Answer from the drawing. Dimensions are ordinates in mm from the lowest x, y and z of the part. A direction names the side the tool comes from. Give positions to 0.01 mm unless a question says otherwise; leave off trailing zeros. Order: outer loops, then holes, each group sorted by start corner. A loop starts at its lowest first (then second) coordinate and runs counter-clockwise, first axis right, second up. Notation, with made-up numbers: (67, 73) - (89, 73) arc R20 ccw to (89, 99) - close; hole circle Ø1 at (29, 25). An arc over 180 degrees is marked (long way). Answer in a Markdown table with one row per item. Add a question column.
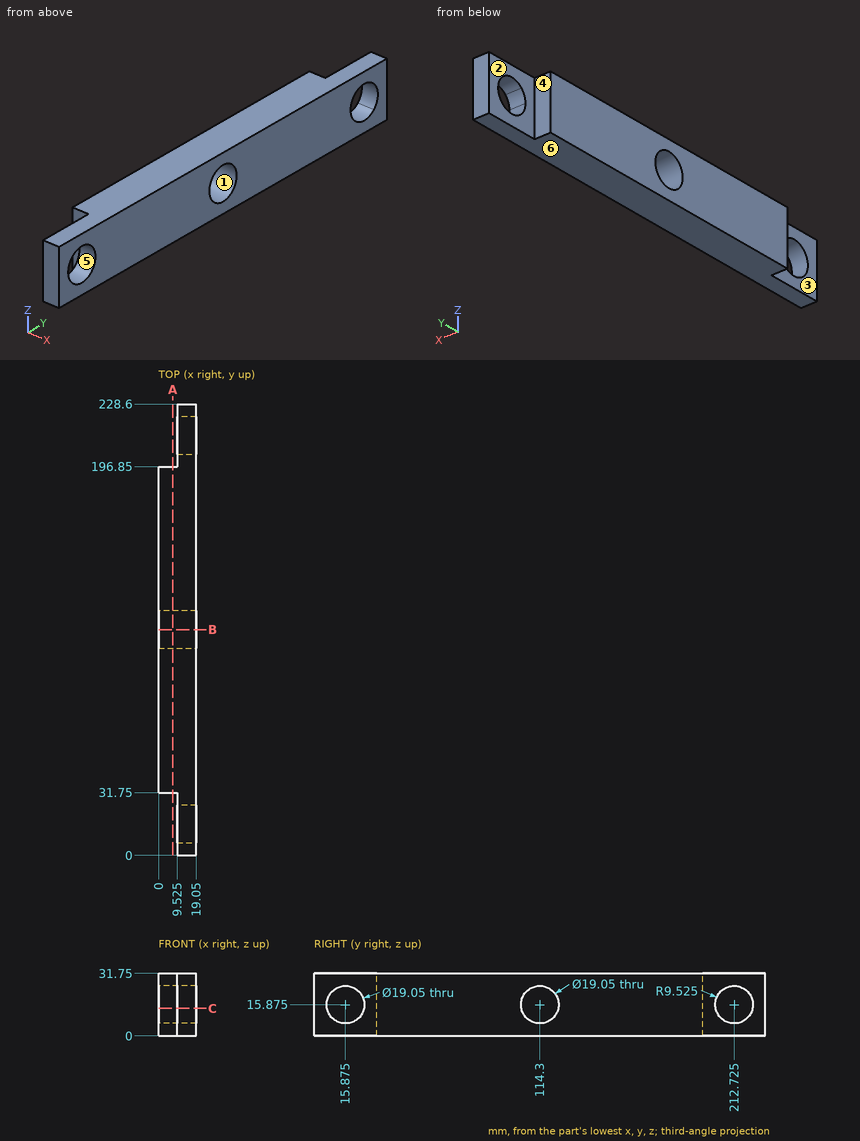
(1) Find section A-A, the plane x = 7.25. Write down the section's boundary in (y, z) (3 decimals), plus the area to 3 significant figures.
(2) Find section C-C, the plane z = 14. Write down the section's boundary in (x, y) (3 decimals), plus the area to 3 significant figures.
(3) The mould has two halves that part along Z. Classify the marked faces 4, 5 and 6: +Z half, -Z half, draft (parallel to the pull), parting line (faces both ways), or undercut.
(4) Straight lines are drawn through the part: line 1 (Z direction, x = 13, y = 114.3); line 2 (Y direction, x = 10.25, z = 8.5); line 3 (X direction, y = 197.5, z = 30) (3 decimals). For each, find the intervals that lie inside material, in ascending order.
(5) Find section B-B, the plane y = 114.3. Write down the section's boundary in (x, z), plus the area to 3 significant figures.
(6) For the marked faces 1, 2 and 3, determine the directions among +Z, -Z, +X, -X, +Y, -Y from which every point of the face is accessible in a straight line to the end or side of a thin tool.
(7) Each of these flat-tipped pins is pushed along its axis until it touches: P1, Ø2, axis at x = 5, z = 12.5, coming from the -Y side; P2, Ø1, axis at x = 2.5, z = 22, coming from the +Y side; P3, Ø6, axis at y = 173.5, z = 14.5, coming from the -X side. Where does it stop, or does it pass through?
Answer key:
| question | item | result |
|---|---|---|
| 1 | outline | (31.75, 0) - (196.85, 0) - (196.85, 31.75) - (31.75, 31.75) - close; hole circle Ø19.05 at (114.3, 15.875) |
| 1 | area | 4,960 mm² |
| 2 | outline | (0, 31.75) - (9.525, 31.75) - (9.525, 25.214) - (19.05, 25.214) - (19.05, 104.961) - (0, 104.961) - close; (0, 123.639) - (19.05, 123.639) - (19.05, 203.386) - (9.525, 203.386) - (9.525, 196.85) - (0, 196.85) - close; (9.525, 0) - (19.05, 0) - (19.05, 6.536) - (9.525, 6.536) - close; (9.525, 222.064) - (19.05, 222.064) - (19.05, 228.6) - (9.525, 228.6) - close |
| 2 | area | 3,040 mm² |
| 3 | face 4 | draft |
| 3 | face 5 | undercut |
| 3 | face 6 | -Z half |
| 4 | line 1 | 0 to 6.35, 25.4 to 31.75 |
| 4 | line 2 | 0 to 9.85, 21.9 to 108.27, 120.33 to 206.7, 218.75 to 228.6 |
| 4 | line 3 | 9.525 to 19.05 |
| 5 | outline | (0, 0) - (19.05, 0) - (19.05, 6.35) - (0, 6.35) - close; (0, 25.4) - (19.05, 25.4) - (19.05, 31.75) - (0, 31.75) - close |
| 5 | area | 242 mm² |
| 6 | face 1 | +X, -X |
| 6 | face 2 | +Z, -Z, -X, +Y |
| 6 | face 3 | +Z, -Z, -X, -Y |
| 7 | P1 | y = 31.75 |
| 7 | P2 | y = 196.85 |
| 7 | P3 | x = 0 |
